The listing builds one solid part. Answer for the finished solid, in the listing's coordinates (mm). Face numbers are marked on the shaded views. A direction names the side the tool comes from. Coordinates: 2 decimals unless noted, no trailing zeros. Write each loop counter-clockwise with the first axis right and the second up, starting at its lowest first coordinate (ties: lowest second). Pieces come first, ordered by that corner, then holes.
(1) Straight lines are drawn through the part: line 1 (X direction, y = -16.75, z = 12.5); line 2 (Y direction, x = 33.5, z = 18.25); line 3 (Y direction, x = 6, z = 10.5). For each, find the intervals that lie inside material, in ascending order.
(2) The part is cut by section C-C on y = -18.25. Determine the outline of the cut face in (x, z).
(3) The part is cut by section A-A on z = 17. Determine the outline of the cut face in (x, y).
(4) Which of the six approach directions +Z, -Z, +X, -X, +Y, -Y give full straight-line access (tool end or side, diameter ignored) to the marked faces 1, 2 and 3?
(5) Given P1, Ø1.5, axis at x = -4, z = 15.5, coming from the +Y side; P2, Ø8, axis at x = 12, z = 16.5, coming from the -Y side, each flat-ended and moving along its own axis, determine where each tip first touches the part or whether it passes through.
(6) For a pull along X with two mould halves and no side action, classify the marked faces 4, 5 and 6 as +X half, -X half, draft (parallel to the pull), parting line (faces both ways), or undercut.
(7) The part is cut by section D-D on x = 19.5. Determine the outline of the cut face in (y, z), plus the area to 3 significant figures.
(8) The part is cut by section B-B on x = 0. Determine the outline of the cut face in (y, z), plus the area to 3 significant figures.
from build123d import *

# Parameters (mm, degrees)
F1_DEPTH = 20
F2_R     = 5
F3_W     = 20
F3_H     = 10
F4_DEPTH = 5
F5_DEPTH = 10
F7_DEPTH = 60.001


with BuildPart() as f1:
    # F0 (on Top) → F1 (new body)
    with BuildSketch(Plane.XY):
        Polygon((17.4899780222, -16.504585755), (17.4899780222, -21.504585755), (37.4899780222, -21.504585755), (37.4899780222, -13.504585755), (-22.5100219778, -13.504585755), (-22.5100219778, -21.504585755), (-2.5100219778, -21.504585755), (-2.5100219778, -16.504585755), align=None)
    extrude(amount=F1_DEPTH)

    # F2
    f2_edges = [f1.edges().sort_by_distance(p)[0] for p in [
        (-22.510022, -17.504586, 0),
        (37.489978, -17.504586, 0),
    ]]
    fillet(f2_edges, radius=F2_R)

    # F3 (on face) → F4 (join)
    with BuildSketch(Plane.XZ.offset(16.504585755)):
        with Locations((7.4899780222, 5)):
            Rectangle(F3_W, F3_H)
    extrude(amount=F4_DEPTH)

    # F5 (add): a face of the model
    f5_faces = [f1.faces().sort_by_distance(p)[0] for p in [
        (7.4899780222, -13.504585755, 10.0801475974),
    ]]
    extrude(f5_faces, amount=F5_DEPTH)

    # F6 (on face) → F7 (cut, through all)
    with BuildSketch(Plane.YZ.offset(37.4899780222)):
        Polygon((-3.504585755, 14.0402622584), (-3.504585755, 20), (-13.504585755, 20), (-13.504585755, 10), align=None)
    extrude(amount=-F7_DEPTH, mode=Mode.SUBTRACT)


solid = f1.part
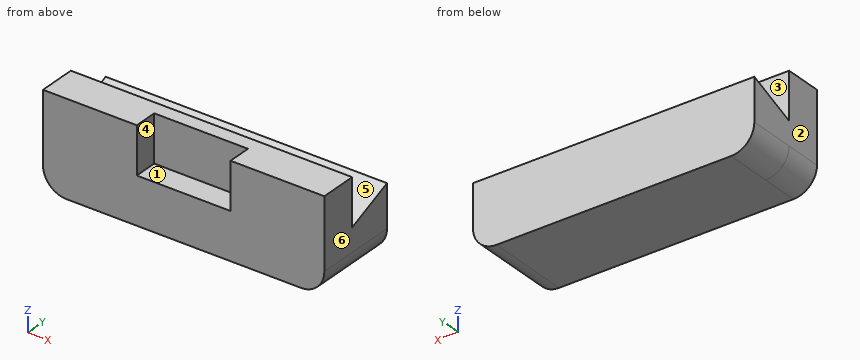
Model answer:
1. line 1: x = -22.51 to -2.51, 17.49 to 37.49
1. line 2: y = -21.5 to -13.5
1. line 3: y = -16.5 to -13.5, -12.27 to -3.5
2. outline: (-22.51, 5) arc R5 ccw to (-17.51, 0) - (32.49, 0) arc R5 ccw to (37.49, 5) - (37.49, 20) - (17.49, 20) - (17.49, 10) - (-2.51, 10) - (-2.51, 20) - (-22.51, 20) - close
3. outline: (-22.51, -21.5) - (-2.51, -21.5) - (-2.51, -16.5) - (17.49, -16.5) - (17.49, -21.5) - (37.49, -21.5) - (37.49, -13.5) - (-22.51, -13.5) - close
4. face 1: +Z, -Y
4. face 2: +Z, -Z, -X, +Y, -Y
4. face 3: +Z, +X, -X
5. P1: stops at y = -13.5
5. P2: stops at y = -16.5
6. face 4: undercut
6. face 5: draft
6. face 6: +X half
7. outline: (-21.5, 0) - (-3.5, 0) - (-3.5, 14.04) - (-13.5, 10) - (-13.5, 20) - (-21.5, 20) - close
7. area: 280 mm2
8. outline: (-21.5, 0) - (-3.5, 0) - (-3.5, 14.04) - (-13.5, 10) - (-13.5, 20) - (-16.5, 20) - (-16.5, 10) - (-21.5, 10) - close
8. area: 230 mm2
